from build123d import *

# Parameters (mm, degrees)
F3_DEPTH    = 5
F4_C1_SIZE2 = 0.3639702343
F4_C1_SIZE  = 1
F4_C2_SIZE2 = 0.3639702343
F4_C2_SIZE  = 1
F4_C3_SIZE2 = 0.3639702343
F4_C3_SIZE  = 1
F4_C4_SIZE2 = 0.3639702343
F4_C4_SIZE  = 1
F4_C5_SIZE2 = 0.3639702343
F4_C5_SIZE  = 1
F4_C6_SIZE2 = 1
F4_C6_SIZE  = 0.3639702343
F4_C7_SIZE2 = 0.3639702343
F4_C7_SIZE  = 1
F4_C8_SIZE2 = 1
F4_C8_SIZE  = 0.3639702343
F4_C9_SIZE2 = 0.3639702343
F4_C9_SIZE  = 1
F5_SIZE     = 0.6
F6_R        = 0.5


with BuildPart() as f1:
    # F0 (on Front) → F1 (revolve)
    with BuildSketch(Plane.XZ):
        Polygon((10.7, 8.5), (0, 8.5), (0, 5), (2, 5), (2, 0), (4, 0), (4, 6), (6, 6), (6, 6.5), (10.7, 6.5), align=None)
    revolve(axis=Axis((0, 0, 6.75), (0, 0, -1)))

    # F2 (on face) → F3 (cut)
    with BuildSketch(Plane(origin=(0, 0, 0), x_dir=(1, 0, 0), z_dir=(0, 0, -1))):
        with BuildLine():
            ThreePointArc((4, 0), (3.4641016151, -2), (2, -3.4641016151))
            Line((2, -3.4641016151), (3, -5.1961524227))
            Line((3, -5.1961524227), (5.9853843016, 0.4185388425))
            Line((5.9853843016, 0.4185388425), (3.990256201, 0.279025895))
            ThreePointArc((3.990256201, 0.279025895), (3.9975633081, 0.1395979868), (4, 0))
        make_face()
        with BuildLine():
            ThreePointArc((-2.2367716139, 3.3161502902), (-0.1395979868, 3.9975633081), (2, 3.4641016151))
            Line((2, 3.4641016151), (3, 5.1961524227))
            Line((3, 5.1961524227), (-3.3551574208, 4.9742254353))
            Line((-3.3551574208, 4.9742254353), (-2.2367716139, 3.3161502902))
        make_face()
        with BuildLine():
            ThreePointArc((-0.8767422936, -1.7975880926), (-1.6960961923, -1.0598385285), (-2, 0))
            Line((-2, 0), (-4, 0))
            ThreePointArc((-4, 0), (-3.3921923846, -2.1196770569), (-1.7534845872, -3.5951761852))
            Line((-1.7534845872, -3.5951761852), (-0.8767422936, -1.7975880926))
        make_face()
        with BuildLine():
            ThreePointArc((-1.7534845872, -3.5951761852), (-3.3921923846, -2.1196770569), (-4, 0))
            Line((-4, 0), (-6, 0))
            Line((-6, 0), (-2.6302268807, -5.3927642778))
            Line((-2.6302268807, -5.3927642778), (-1.7534845872, -3.5951761852))
        make_face()
        with BuildLine():
            ThreePointArc((2, 0), (1.7320508076, -1), (1, -1.7320508076))
            Line((1, -1.7320508076), (2, -3.4641016151))
            ThreePointArc((2, -3.4641016151), (3.4641016151, -2), (4, 0))
            ThreePointArc((4, 0), (3.9975633081, 0.1395979868), (3.990256201, 0.279025895))
            Line((3.990256201, 0.279025895), (1.9951281005, 0.1395129475))
            ThreePointArc((1.9951281005, 0.1395129475), (1.998781654, 0.0697989934), (2, 0))
        make_face()
        with BuildLine():
            ThreePointArc((-1.1183858069, 1.6580751451), (-0.0697989934, 1.998781654), (1, 1.7320508076))
            Line((1, 1.7320508076), (2, 3.4641016151))
            ThreePointArc((2, 3.4641016151), (-0.1395979868, 3.9975633081), (-2.2367716139, 3.3161502902))
            Line((-2.2367716139, 3.3161502902), (-1.1183858069, 1.6580751451))
        make_face()
        with BuildLine():
            ThreePointArc((-0.4983586629, -1.0217866811), (-0.9640965616, -0.6024343936), (-1.1368418442, 0))
            Line((-1.1368418442, 0), (-2, 0))
            ThreePointArc((-2, 0), (-1.6960961923, -1.0598385285), (-0.8767422936, -1.7975880926))
            Line((-0.8767422936, -1.7975880926), (-0.4983586629, -1.0217866811))
        make_face()
        with BuildLine():
            Line((-0.4983586629, -1.0217866811), (0, 0))
            Line((0, 0), (-1.1368418442, 0))
            ThreePointArc((-1.1368418442, 0), (-0.9640965616, -0.6024343936), (-0.4983586629, -1.0217866811))
        make_face()
        with BuildLine():
            Line((-0.6357138916, 0.9424846029), (0, 0))
            Line((0, 0), (0.5684209221, 0.9845339171))
            ThreePointArc((0.5684209221, 0.9845339171), (-0.0396752082, 1.1361493108), (-0.6357138916, 0.9424846029))
        make_face()
        with BuildLine():
            ThreePointArc((-0.6357138916, 0.9424846029), (-0.0396752082, 1.1361493108), (0.5684209221, 0.9845339171))
            Line((0.5684209221, 0.9845339171), (1, 1.7320508076))
            ThreePointArc((1, 1.7320508076), (-0.0697989934, 1.998781654), (-1.1183858069, 1.6580751451))
            Line((-1.1183858069, 1.6580751451), (-0.6357138916, 0.9424846029))
        make_face()
        with BuildLine():
            Line((1.1340725546, 0.0793020783), (0, 0))
            Line((0, 0), (0.5684209221, -0.9845339171))
            ThreePointArc((0.5684209221, -0.9845339171), (0.9845339171, -0.5684209221), (1.1368418442, 0))
            ThreePointArc((1.1368418442, 0), (1.1361493108, 0.0396752082), (1.1340725546, 0.0793020783))
        make_face()
        with BuildLine():
            ThreePointArc((1.1368418442, 0), (0.9845339171, -0.5684209221), (0.5684209221, -0.9845339171))
            Line((0.5684209221, -0.9845339171), (1, -1.7320508076))
            ThreePointArc((1, -1.7320508076), (1.7320508076, -1), (2, 0))
            ThreePointArc((2, 0), (1.998781654, 0.0697989934), (1.9951281005, 0.1395129475))
            Line((1.9951281005, 0.1395129475), (1.1340725546, 0.0793020783))
            ThreePointArc((1.1340725546, 0.0793020783), (1.1361493108, 0.0396752082), (1.1368418442, 0))
        make_face()
    extrude(amount=-F3_DEPTH, mode=Mode.SUBTRACT)

    # F4: chamfer of 1 x 0.3639702343 on 9 edges, made by hand

    # F4_c1
    f4_c1_edges = [f1.edges().sort_by_distance(p)[0] for p in [
        (0.1395979868, 3.9975633081, 0),
    ]]
    f4_c1_side = f1.faces().sort_by_distance((0.1395979868, 3.9975633081, 0.0072794047))[0]
    chamfer(f4_c1_edges, length=F4_C1_SIZE, length2=F4_C1_SIZE2, reference=f4_c1_side)

    # F4_c2
    f4_c2_edges = [f1.edges().sort_by_distance(p)[0] for p in [
        (-3.5317903714, -1.8778862511, 0),
    ]]
    f4_c2_side = f1.faces().sort_by_distance((-3.5317903714, -1.8778862511, 0.0072794047))[0]
    chamfer(f4_c2_edges, length=F4_C2_SIZE, length2=F4_C2_SIZE2, reference=f4_c2_side)

    # F4_c3
    f4_c3_edges = [f1.edges().sort_by_distance(p)[0] for p in [
        (3.3921923846, -2.1196770569, 0),
    ]]
    f4_c3_side = f1.faces().sort_by_distance((3.3921923846, -2.1196770569, 0.0072794047))[0]
    chamfer(f4_c3_edges, length=F4_C3_SIZE, length2=F4_C3_SIZE2, reference=f4_c3_side)

    # F4_c4
    f4_c4_edges = [f1.edges().sort_by_distance(p)[0] for p in [
        (2.8111503402, -0.1965747812, 0),
    ]]
    f4_c4_side = f1.faces().sort_by_distance((2.8111503402, -0.1965747812, 0.0072794047))[0]
    chamfer(f4_c4_edges, length=F4_C4_SIZE, length2=F4_C4_SIZE2, reference=f4_c4_side)

    # F4_c5
    f4_c5_edges = [f1.edges().sort_by_distance(p)[0] for p in [
        (1.4090074414, 2.4404724768, 0),
    ]]
    f4_c5_side = f1.faces().sort_by_distance((1.4090074414, 2.4404724768, 0.0072794047))[0]
    chamfer(f4_c5_edges, length=F4_C5_SIZE, length2=F4_C5_SIZE2, reference=f4_c5_side)

    # F4_c6
    f4_c6_edges = [f1.edges().sort_by_distance(p)[0] for p in [
        (-1.2353364159, 2.5328149991, 0),
    ]]
    f4_c6_side = f1.faces().sort_by_distance((-1.2287937303, 2.5360060801, 0))[0]
    chamfer(f4_c6_edges, length=F4_C6_SIZE, length2=F4_C6_SIZE2, reference=f4_c6_side)

    # F4_c7
    f4_c7_edges = [f1.edges().sort_by_distance(p)[0] for p in [
        (-2.8180148829, 0, 0),
    ]]
    f4_c7_side = f1.faces().sort_by_distance((-2.8180148829, 0, 0.0072794047))[0]
    chamfer(f4_c7_edges, length=F4_C7_SIZE, length2=F4_C7_SIZE2, reference=f4_c7_side)

    # F4_c8
    f4_c8_edges = [f1.edges().sort_by_distance(p)[0] for p in [
        (-1.5758139244, -2.3362402179, 0),
    ]]
    f4_c8_side = f1.faces().sort_by_distance((-1.5818488244, -2.3321696265, 0))[0]
    chamfer(f4_c8_edges, length=F4_C8_SIZE, length2=F4_C8_SIZE2, reference=f4_c8_side)

    # F4_c9
    f4_c9_edges = [f1.edges().sort_by_distance(p)[0] for p in [
        (1.4090074414, -2.4404724768, 0),
    ]]
    f4_c9_side = f1.faces().sort_by_distance((1.4090074414, -2.4404724768, 0.0072794047))[0]
    chamfer(f4_c9_edges, length=F4_C9_SIZE, length2=F4_C9_SIZE2, reference=f4_c9_side)

    # F5
    f5_edges = [f1.edges().sort_by_distance(p)[0] for p in [
        (-10.7, 0, 8.5),
        (-10.7, 0, 6.5),
    ]]
    chamfer(f5_edges, length=F5_SIZE)

    # F6
    f6_edges = [f1.edges().sort_by_distance(p)[0] for p in [
        (10.7, 0, 7.5),
        (-10.7, 0, 7.1),
        (-10.7, 0, 7.9),
    ]]
    fillet(f6_edges, radius=F6_R)


solid = f1.part
Geometry: final body of the model. Coordinates: model frame, mm. A direction names the side the tool comes from. Coordinates: 2 decimals unless noted, no trailing zeros. Order: outer loops, then holes, each group sorted by start corner. A loop starts at its lowest first (then second) coordinate and runs counter-clockwise, first axis right, second up.
(1) Material intervals for probe 1 along Z at (x, y) = (-5, -5.25); probe 2 along Z at (x, y) = (-5, 1); probe 3 along X at (y, z) = (-1, 1.75), sorted ascending.
(2) Access query for faces 1 (the face through (0, 0, 5)), 2 (the face through (3.01, -0.21, 2.97)), 3 (the face through (1.5, -2.6, 3)), 4 (the face through (-3, 0, 3)). Directions: +Z, -Z, +X, -X, +Y, -Y. A direction counts if a zero-diameter tool reaches every point of the face in a straight line with its end or side. Return the directions, or none.
(3) First-contact query: pin 1 (1.5 mm diameter, centred on y = 2.5, z = 5.5, fed in from +X); pin 2 (10 mm diameter, centred on x = 8, y = 0.5, fed in from -Z); pin 3 (2 mm diameter, centred on x = -2.5, z = 2.5, fed in from +Y); pin 4 (3 mm diameter, centred on y = -6.5, z = 4, fed in from +X). Flat tips, straight axial feed; report the tip coordinate or a pass-through.
(4) Section query A-A (z = 4.25). Return the cut outline in (x, y).
(5) Draft query along Y for faces 5 (the face through (9.884, 4.098, 7.503)), 6 (the face through (2.977, -0.393, 0.493)), 7 (the face through (1.32, 2.66, 0.49)). Return one class per face: pulls with the +Y half, pulls with the -Y half, needs draft (parallel to the pull), parting line crosses it, or undercut.
Solution:
1. probe 1: z = 6.5 to 8.5
1. probe 2: z = 6 to 8.5
1. probe 3: x = -3.87 to -1.73, 1.73 to 3.87
2. face 1: -Z
2. face 2: -Z, +X, +Y
2. face 3: -Z, -Y
2. face 4: -Z, +X, -X, +Y
3. pin 1: stops at x = 5.68
3. pin 2: stops at z = 0
3. pin 3: stops at y = 3.71
3. pin 4: passes through
4. outline: (-4, 0) arc R4 ccw to (-2.24, -3.32) - (-1.12, -1.66) arc R2 cw to (-2, 0) - close; (-1.75, 3.6) - (-0.88, 1.8) arc R2 cw to (1, 1.73) - (2, 3.46) arc R4 ccw to start; (1, -1.73) - (2, -3.46) arc R4 ccw to (3.99, -0.28) - (2, -0.14) arc R2 cw to start
5. face 5: parting line crosses it
5. face 6: pulls with the +Y half
5. face 7: undercut
